from build123d import *

# Parameters (mm, degrees)
CYLINDER026_R           = 1.6
CYLINDER026_DEPTH       = 10
CYLINDER026_PITCH_ANGLE = 90
BOX008_W                = 17
BOX008_H                = 10
BOX008_DEPTH            = 5
BOX019_W                = 6
BOX019_H                = 16
BOX019_DEPTH            = 3
BOX007_W                = 17
BOX007_H                = 13
BOX007_DEPTH            = 10
BOX002_W                = 3
BOX002_H                = 85
BOX002_DEPTH            = 30


with BuildPart() as front_hole:
    # Cylinder026 → Cylinder026 (new body)
    with BuildSketch(Plane.XY):
        Circle(CYLINDER026_R)
    extrude(amount=CYLINDER026_DEPTH)


with BuildPart() as front_hole_1:
    # Cylinder026 pitch: moved
    add(front_hole.part.rotate(Axis((0, 0, 0), (0, 1, 0)), CYLINDER026_PITCH_ANGLE))


with BuildPart() as front_hole_2:
    # Cylinder026 placement: moved
    add(front_hole_1.part.moved(Location((-7.4, 38.69, -18.9))))


with BuildPart() as usb_connector002:
    # Box008 → Box008 (new body)
    with BuildSketch(Plane(origin=(-11, 49, -16), x_dir=(1, 0, 0), z_dir=(0, 0, 1))):
        with Locations((8.5, 5)):
            Rectangle(BOX008_W, BOX008_H)
    extrude(amount=BOX008_DEPTH)


with BuildPart() as sd_card_reader:
    # Box019 → Box019 (new body)
    with BuildSketch(Plane(origin=(-8, 42, -4), x_dir=(1, 0, 0), z_dir=(0, 0, 1))):
        with Locations((3, 8)):
            Rectangle(BOX019_W, BOX019_H)
    extrude(amount=BOX019_DEPTH)


with BuildPart() as fusion:
    # Box007 → Box007 (new body)
    with BuildSketch(Plane(origin=(-11, 20.5, 0), x_dir=(1, 0, 0), z_dir=(0, 0, 1))):
        with Locations((8.5, 6.5)):
            Rectangle(BOX007_W, BOX007_H)
    extrude(amount=BOX007_DEPTH)

    # Fusion: union USB connector002, SD card reader
    add(usb_connector002.part)
    add(sd_card_reader.part)


with BuildPart() as final_front:
    # Box002 → Box002 (new body)
    with BuildSketch(Plane(origin=(-5, 0, -25), x_dir=(1, 0, 0), z_dir=(0, 0, 1))):
        with Locations((1.5, 42.5)):
            Rectangle(BOX002_W, BOX002_H)
    extrude(amount=BOX002_DEPTH)

    # Cut: cut Fusion
    add(fusion.part, mode=Mode.SUBTRACT)

    # Cut027: cut front hole
    add(front_hole_2.part, mode=Mode.SUBTRACT)


solid = final_front.part
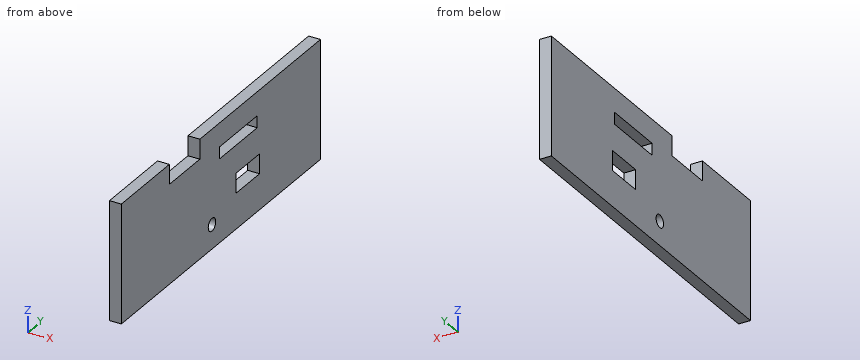
Verification items for the finished model (mm, model axes). Coordinates: 2 decimals unless noted, no trailing zeros. Order: outer loops, then holes, each group sorted by start corner. A loop starts at its lowest first (then second) coordinate and runs counter-clockwise, first axis right, second up.
Item 1: Section check A-A, the plane y = 38.69. Enter the section's corners in (x, z).
Filled in:
outline: (-5, -25) - (-2, -25) - (-2, -20.5) - (-5, -20.5) - close; (-5, -17.3) - (-2, -17.3) - (-2, 5) - (-5, 5) - close
Item 2: Section check B-B, the plane z = -18.9. Enter the section's corners in (x, y).
Filled in:
outline: (-5, 0) - (-2, 0) - (-2, 37.09) - (-5, 37.09) - close; (-5, 40.29) - (-2, 40.29) - (-2, 85) - (-5, 85) - close
Item 3: Section check D-D, the plane x = -3. Enter the section's corners in (y, z).
Filled in:
outline: (0, -25) - (85, -25) - (85, 5) - (33.5, 5) - (33.5, 0) - (20.5, 0) - (20.5, 5) - (0, 5) - close; hole circle Ø3.2 at (38.69, -18.9); hole (42, -4) - (58, -4) - (58, -1) - (42, -1) - close; hole (49, -16) - (59, -16) - (59, -11) - (49, -11) - close
Item 4: Material ranges on L1, parallel to Y at x = -4.3, z = -14.5; L2, parallel to Y at x = -3.95, z = -18.9; L3, parallel to Z at x = -2.95, y = 38.69, recorded low to high.
Filled in:
L1: y = 0 to 49, 59 to 85
L2: y = 0 to 37.09, 40.29 to 85
L3: z = -25 to -20.5, -17.3 to 5
Item 5: Depth check by flat-ended pin: pin 1 (5 mm diameter, centred on y = 38.69, z = -18.9, fed in from -X). Enter the tip coordinate at first touch or a pass-through.
Filled in:
pin 1: stops at x = -5
Item 6: Section check C-C, the plane y = 51.5. Enter the section's corners in (x, z), then the cut area to 3 significant figures.
Filled in:
outline: (-5, -25) - (-2, -25) - (-2, -16) - (-5, -16) - close; (-5, -11) - (-2, -11) - (-2, -4) - (-5, -4) - close; (-5, -1) - (-2, -1) - (-2, 5) - (-5, 5) - close
area: 66.0 mm2
